The listing builds one solid part. Answer for the finished solid, in the listing's coordinates (mm). A direction names the side the tool comes from. Coordinates: 2 decimals unless noted, no trailing zeros. Write each loop counter-clockwise with the first axis right and the second up, starting at its lowest first coordinate (ties: lowest second). Pieces come first, ordered by that corner, then holes. Notation, with made-up numbers: M 23,-34 L 47,-34 A13 ccw 47,-15 Z; hole C 3,16 d3. An arc over 180 degrees is marked long. Put each result on its own line as item: value. Start each with the question number.
```python
from build123d import *

# Parameters (mm, degrees)
SKETCH_W        = 61.5
SKETCH_H        = 61.5
PAD_DEPTH       = 8
SKETCH001_R     = 1.5
POCKET_DEPTH    = 6
SKETCH002_W     = 61.5
SKETCH002_H     = 61.5
SKETCH002_W_2   = 57.5
SKETCH002_H_2   = 57.5
POCKET001_DEPTH = 2
SKETCH003_W     = 55.5
SKETCH003_H     = 55.5
POCKET002_DEPTH = 2
FILLET_R        = 4
FILLET001_R     = 3
SKETCH004_W     = 20
SKETCH004_H     = 35
POCKET003_DEPTH = 1
POCKET004_DEPTH = 4
FILLET002_R     = 2
FILLET003_R     = 4
FILLET004_R     = 1.8


with BuildPart() as part:
    # Sketch → Pad (new body)
    with BuildSketch(Plane.XY):
        Rectangle(SKETCH_W, SKETCH_H)
    extrude(amount=PAD_DEPTH)

    # Sketch001 (on Face6 of Pad) → Pocket (cut)
    with BuildSketch(Plane.XY.offset(8)):
        with Locations((-24, 0)):
            Circle(SKETCH001_R)
        with Locations((24, 0)):
            Circle(SKETCH001_R)
        Polygon((-10, 8.25), (10, 8.25), (10, -26.75), (4.5, -26.75), (4.5, -30.75), (-4.5, -30.75), (-4.5, -26.75), (-10, -26.75), align=None)
    extrude(amount=-POCKET_DEPTH, mode=Mode.SUBTRACT)

    # Sketch002 (on Face5 of Pocket) → Pocket001 (cut)
    with BuildSketch(Plane.XY.offset(8)):
        Rectangle(SKETCH002_W, SKETCH002_H)
        Rectangle(SKETCH002_W_2, SKETCH002_H_2, mode=Mode.SUBTRACT)
    extrude(amount=-POCKET001_DEPTH, mode=Mode.SUBTRACT)

    # Sketch003 (on Face15 of Pocket001) → Pocket002 (cut)
    with BuildSketch(Plane.XY.offset(8)):
        Rectangle(SKETCH003_W, SKETCH003_H)
    extrude(amount=-POCKET002_DEPTH, mode=Mode.SUBTRACT)

    # Fillet
    fillet_edges = [part.edges().sort_by_distance(p)[0] for p in [
        (-30.75, -30.75, 3),
        (30.75, -30.75, 3),
        (-30.75, 30.75, 3),
        (30.75, 30.75, 3),
    ]]
    fillet(fillet_edges, radius=FILLET_R)

    # Fillet001
    fillet001_edges = [part.edges().sort_by_distance(p)[0] for p in [
        (28.75, -28.75, 7),
        (28.75, 28.75, 7),
        (-28.75, -28.75, 7),
        (-28.75, 28.75, 7),
        (27.75, 27.75, 7),
        (-27.75, 27.75, 7),
        (-27.75, -27.75, 7),
        (27.75, -27.75, 7),
    ]]
    fillet(fillet001_edges, radius=FILLET001_R)

    # Sketch004 (on Face25 of Fillet001) → Pocket003 (cut)
    with BuildSketch(Plane.XY.offset(2)):
        with Locations((0, -9.25)):
            Rectangle(SKETCH004_W, SKETCH004_H)
    extrude(amount=-POCKET003_DEPTH, mode=Mode.SUBTRACT)

    # Sketch005 (on Face23 of Pocket003) → Pocket004 (cut)
    with BuildSketch(Plane.XY.offset(6)):
        with BuildLine():
            Line((-26.5, 26.459332), (26.5, 26.459332))
            Line((26.5, 26.459332), (26.5, 6))
            ThreePointArc((26.5, 6), (20.5, 0), (26.5, -6))
            Line((26.5, -6), (26.5, -26.540668))
            Line((26.5, -26.540668), (13, -26.540668))
            Line((13, -26.540668), (13, 11.25))
            Line((-13, 11.25), (13, 11.25))
            Line((-13, 11.25), (-13, -26.540668))
            Line((-13, -26.540668), (-26.5, -26.540668))
            Line((-26.5, -26.540668), (-26.5, -6))
            ThreePointArc((-26.5, -6), (-20.5, 0), (-26.5, 6))
            Line((-26.5, 6), (-26.5, 26.459332))
        make_face()
    extrude(amount=-POCKET004_DEPTH, mode=Mode.SUBTRACT)

    # Fillet002
    fillet002_edges = [part.edges().sort_by_distance(p)[0] for p in [
        (-26.5, 26.459332, 4),
        (26.5, 26.459332, 4),
        (-26.5, -26.540668, 4),
        (26.5, -26.540668, 4),
        (-13, -26.540668, 4),
        (13, -26.540668, 4),
    ]]
    fillet(fillet002_edges, radius=FILLET002_R)

    # Fillet003
    fillet003_edges = [part.edges().sort_by_distance(p)[0] for p in [
        (13, 11.25, 4),
        (-13, 11.25, 4),
    ]]
    fillet(fillet003_edges, radius=FILLET003_R)

    # Fillet004
    fillet004_edges = [part.edges().sort_by_distance(p)[0] for p in [
        (0, 30.75, 0),
        (-29.578427, 29.578427, 0),
        (29.578427, 29.578427, 0),
        (-30.75, 0, 0),
        (30.75, 0, 0),
        (-29.578427, -29.578427, 0),
        (29.578427, -29.578427, 0),
        (0, -30.75, 0),
    ]]
    fillet(fillet004_edges, radius=FILLET004_R)


solid = part.part
```
1) Determine the mould class of faces 1 (the face through (-26.85, -26.89, 6.99)), 2 (the face through (-28, 13, 8)), 3 (the face through (-27.85, -27.89, 6.99)) for opening direction X: +X half, -X half, draft (parallel to the pull), parting line (faces both ways), or undercut.
2) A cutting plane is placed at C-C on y = 23. Write down the section's boundary in (x, z), then the cut area to 3 significant figures.
3) Given pin 1 Ø1.5 at (x, y) = (24, 0) entering from +Z; pin 2 Ø0.6 at (x, z) = (2, 7) entering from -Y; pin 3 Ø1.2 at (y, z) = (-28, 4) entering from -X, each flat-ended and moving along its own axis, determine where each tip first touches the part or whether it passes through.
4) A cutting plane is placed at D-D on x = 7.5. Write down the section's boundary in (y, z), then the cut area to 3 significant figures.
5) Straight lines are drawn through the part: probe 1 along X at (y, z) = (-21, 4); probe 2 along Y at (x, z) = (-8.5, 5.25); probe 3 along Y at (x, z) = (0, 4.25). For each, find the intervals that lie inside material, in ascending order.
6) For faces 4 (the face through (-26.5, -15, 4)), 5 (the face through (-29.609, -29.547, 3.929)), 6 (the face through (4.5, -29, 4)), determine the directions among +Z, -Z, +X, -X, +Y, -Y from which every point of the face is accessible in a straight line to the end or side of a thin tool.
7) A cutting plane is placed at B-B on x = 16. Write down the section's boundary in (y, z).
Answers follow:
1. face 1: undercut
1. face 2: draft
1. face 3: -X half
2. outline: M -30.75,1.8 A1.8 ccw -28.95,0 L 28.95,0 A1.8 ccw 30.75,1.8 L 30.75,6 L 28.75,6 L 28.75,8 L 27.75,8 L 27.75,6 L 26.5,6 L 26.5,2 L -26.5,2 L -26.5,6 L -27.75,6 L -27.75,8 L -28.75,8 L -28.75,6 L -30.75,6 Z
2. area: 160 mm²
3. pin 1: stops at z = 2
3. pin 2: stops at y = 27.75
3. pin 3: stops at x = -30.7
4. outline: M -30.75,1.8 A1.8 ccw -28.95,0 L 28.95,0 A1.8 ccw 30.75,1.8 L 30.75,6 L 28.75,6 L 28.75,8 L 27.75,8 L 27.75,6 L 26.46,6 L 26.46,2 L 11.25,2 L 11.25,6 L 8.25,6 L 8.25,1 L -26.75,1 L -26.75,6 L -27.75,6 L -27.75,8 L -28.75,8 L -28.75,6 L -30.75,6 Z
4. area: 136 mm²
5. probe 1: x = -30.75 to -26.5, -13 to -10, 10 to 13, 26.5 to 30.75
5. probe 2: y = -30.75 to -26.75, 8.25 to 11.25, 26.46 to 30.75
5. probe 3: y = 8.25 to 11.25, 26.46 to 30.75
6. face 4: +Z
6. face 5: +Z, -Z, -X, -Y
6. face 6: +Z, -Y
7. outline: M -30.75,1.8 A1.8 ccw -28.95,0 L 28.95,0 A1.8 ccw 30.75,1.8 L 30.75,6 L 28.75,6 L 28.75,8 L 27.75,8 L 27.75,6 L 26.46,6 L 26.46,2 L -26.54,2 L -26.54,6 L -27.75,6 L -27.75,8 L -28.75,8 L -28.75,6 L -30.75,6 Z
